Here's the drawing with two shaded views (mm, measured from the low corner). I have some questions. Round coordinates to 2 decimals unless told otherwise and drop trailing zeros. Loops run counter-clockwise (first coordinate to the right, second up) from the corner with the lowest first, then second, coordinate; pieces in that order, holes last. Notation, with made-up numbers: M 14.25,45 L 40.25,45 A15 ccw 40.25,61 Z; hole C 60,-18 d1. An arc over 180 degrees is marked long. Answer as a JSON object with one key per item and string values.
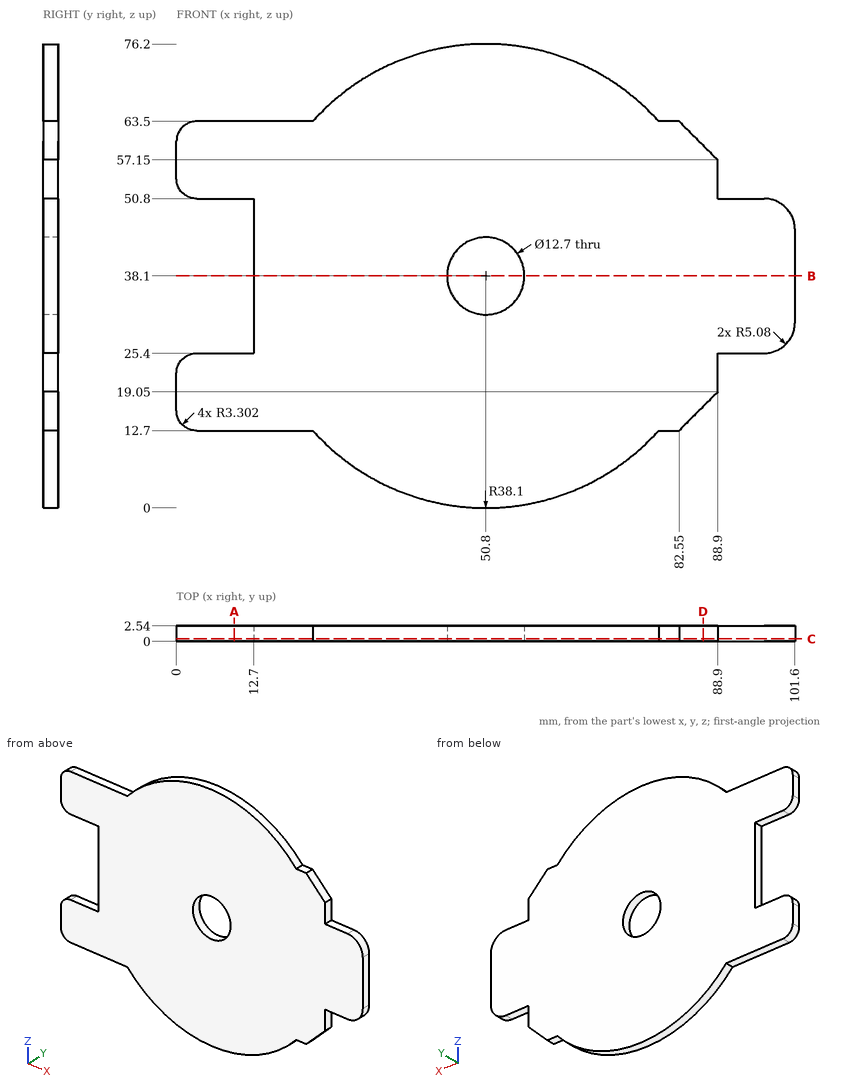
Item 1: I want a section at B-B on z = 38.1. List the corners of the cut face in (x, y) for me.
Solution:
{"outline": "M 12.7,0 L 44.45,0 L 44.45,2.54 L 12.7,2.54 Z; M 57.15,0 L 101.6,0 L 101.6,2.54 L 57.15,2.54 Z"}
Item 2: I want a section at C-C on y = 0.4. List the corners of the cut face in (x, z) for me.
Solution:
{"outline": "M 0,16 A3.3 ccw 3.3,12.7 L 22.4,12.7 A38.1 ccw 79.2,12.7 L 82.55,12.7 L 88.9,19.05 L 88.9,25.4 L 96.52,25.4 A5.08 ccw 101.6,30.48 L 101.6,45.72 A5.08 ccw 96.52,50.8 L 88.9,50.8 L 88.9,57.15 L 82.55,63.5 L 79.2,63.5 A38.1 ccw 22.4,63.5 L 3.3,63.5 A3.3 ccw 0,60.2 L 0,54.1 A3.3 ccw 3.3,50.8 L 12.7,50.8 L 12.7,25.4 L 3.3,25.4 A3.3 ccw 0,22.1 Z; hole C 50.8,38.1 d12.7"}
Item 3: I want a section at D-D on x = 86.5. List the corners of the cut face in (y, z) for me, plus the area to 3 significant figures.
Solution:
{"outline": "M 0,16.65 L 2.54,16.65 L 2.54,59.55 L 0,59.55 Z", "area": "109 mm2"}
Item 4: For P1, Ø0.8, axis at y = 1.5, z = 22.5, coming from the +X side; P2, Ø0.8, axis at y = 1, z = 41, coming from the -X side; P3, Ø1.5, axis at x = 65, y = 1.5, coming from the +Z side, each with a flat end and sliding along its axis, tell me the tip position at first contact or that it passes through.
Solution:
{"P1": "stops at x = 88.9", "P2": "stops at x = 12.7", "P3": "stops at z = 73.75"}
Item 5: If I drill on L1, parallel to Z at x = 50.8, y = 1.9; L2, parallel to Z at x = 14.5, y = 2.4; L3, parallel to X at y = 2.15, z = 36, over which ranges is the centre line in solid material (lowest first)? Write a range as from..to.
Solution:
{"L1": "z = 0..31.75, 44.45..76.2", "L2": "z = 12.7..63.5", "L3": "x = 12.7..44.81, 56.79..101.6"}
Item 6: I want a section at A-A on x = 9.5. List the corners of the cut face in (y, z) for me.
Solution:
{"outline": "M 0,12.7 L 2.54,12.7 L 2.54,25.4 L 0,25.4 Z; M 0,50.8 L 2.54,50.8 L 2.54,63.5 L 0,63.5 Z"}
